```python
from build123d import *

# Parameters (mm, degrees)
SKETCH3_W           = 2.234278516
SKETCH3_H           = 3.869883908
BOSS_EXTRUDE1_DEPTH = 3.81
SKETCH4_W           = 2.234278516
SKETCH4_H           = 3.81
BOSS_EXTRUDE2_DEPTH = 1.27
SKETCH7_W           = 2.234278516
SKETCH7_H           = 3.81
BOSS_EXTRUDE3_DEPTH = 1.27
CUT_EXTRUDE3_DEPTH  = 2.286
FILLET1_R           = 0.254


with BuildPart() as part:
    # Sketch1 → Revolve1 (revolve)
    with BuildSketch(Plane.XY):
        with BuildLine():
            Line((0, 0), (6.604, 0))
            Line((6.604, 0), (6.604, 1.524))
            Line((6.604, 1.524), (5.526369265, 2.601630735))
            ThreePointArc((5.526369265, 2.601630735), (5.623645794, 3.729450681), (5.02050731, 4.687398762))
            Line((5.02050731, 4.687398762), (5.02050731, 6.211398762))
            add(Edge.make_bspline(
                [(5.02050731, 6.211398762), (2.796634976, 16.191993282), (2.733543957, 26.472012216)],
                knots=[0, 0, 0, 1, 1, 1], degree=2))
            Line((2.733543957, 26.472012216), (2.733543957, 31.552012216))
            ThreePointArc((2.733543957, 31.552012216), (3.551212648, 32.965759778), (2.300394609, 34.015863816))
            Line((2.300394609, 34.015863816), (2.300394609, 34.777863816))
            ThreePointArc((2.300394609, 34.777863816), (2.528411489, 35.490223347), (2.037352116, 36.054411694))
            add(Edge.make_bspline(
                [(2.037352116, 36.054411694), (2.754588802, 37.690610821), (3.171523279, 39.41712427), (3.279734912, 41.196512193)],
                knots=[0, 0, 0, 0, 0.825528863, 0.825528863, 0.825528863, 0.825528863], degree=3))
            ThreePointArc((3.279734912, 41.196512193), (3.026614336, 42.224230944), (2.234278516, 42.926))
            Line((2.234278516, 42.926), (0, 42.926))
            Line((0, 42.926), (0, 0))
        make_face()
    revolve(axis=Axis((0, 0, 0), (0, 1, 0)))

    # Sketch3 → Boss-Extrude1 (add)
    with BuildSketch(Plane(origin=(0, 42.926, 0), x_dir=(1, 0, 0), z_dir=(0, 1, 0))):
        Rectangle(SKETCH3_W, SKETCH3_H)
    extrude(amount=BOSS_EXTRUDE1_DEPTH)

    # Sketch4 → Boss-Extrude2 (add)
    with BuildSketch(Plane(origin=(0, 0, -1.934941954), x_dir=(-1, 0, 0), z_dir=(0, 0, -1))):
        with Locations((0, 44.831)):
            Rectangle(SKETCH4_W, SKETCH4_H)
    extrude(amount=BOSS_EXTRUDE2_DEPTH)

    # Sketch7 → Boss-Extrude3 (add)
    with BuildSketch(Plane.XY.offset(1.934941954)):
        with Locations((0, 44.831)):
            Rectangle(SKETCH7_W, SKETCH7_H)
    extrude(amount=BOSS_EXTRUDE3_DEPTH)

    # Sketch11 → Cut-Extrude3 (cut)
    with BuildSketch(Plane(origin=(1.117139258, 0, 0), x_dir=(0, 0, -1), z_dir=(1, 0, 0))):
        with BuildLine():
            Line((-1.934941954, 42.926), (-1.33813329, 42.926))
            Line((-1.33813329, 42.926), (-1.33813329, 43.942))
            ThreePointArc((-1.33813329, 43.942), (-1.412528167, 44.121605122), (-1.59213329, 44.196))
            Line((-1.59213329, 44.196), (-2.60813329, 44.196))
            ThreePointArc((-2.60813329, 44.196), (-2.787738412, 44.270394878), (-2.86213329, 44.45))
            Line((-2.86213329, 44.45), (-2.86213329, 45.212))
            ThreePointArc((-2.86213329, 45.212), (-2.787738412, 45.391605122), (-2.60813329, 45.466))
            Line((-2.60813329, 45.466), (-1.59213329, 45.466))
            ThreePointArc((-1.59213329, 45.466), (-1.412528167, 45.540394878), (-1.33813329, 45.72))
            Line((-1.33813329, 45.72), (-1.33813329, 46.10618983))
            Line((-1.33813329, 46.10618983), (-0.180981014, 46.680037288))
            ThreePointArc((-0.180981014, 46.680037288), (-0.06813329, 46.706482039), (0.044714435, 46.680037288))
            Line((0.044714435, 46.680037288), (1.20186671, 46.10618983))
            Line((1.20186671, 46.10618983), (1.20186671, 45.72))
            ThreePointArc((1.20186671, 45.72), (1.276261588, 45.540394878), (1.45586671, 45.466))
            Line((1.45586671, 45.466), (2.47186671, 45.466))
            ThreePointArc((2.47186671, 45.466), (2.651471833, 45.391605122), (2.72586671, 45.212))
            Line((2.72586671, 45.212), (2.72586671, 44.45))
            ThreePointArc((2.72586671, 44.45), (2.651471833, 44.270394878), (2.47186671, 44.196))
            Line((2.47186671, 44.196), (1.45586671, 44.196))
            ThreePointArc((1.45586671, 44.196), (1.276261588, 44.121605122), (1.20186671, 43.942))
            Line((1.20186671, 43.942), (1.20186671, 42.926))
            Line((1.20186671, 42.926), (1.934941954, 42.926))
            Line((1.934941954, 42.926), (3.204941954, 42.926))
            Line((3.204941954, 42.926), (3.204941954, 46.736))
            Line((3.204941954, 46.736), (-3.204941954, 46.736))
            Line((-3.204941954, 46.736), (-3.204941954, 42.926))
            Line((-3.204941954, 42.926), (-1.934941954, 42.926))
        make_face()
    extrude(amount=-CUT_EXTRUDE3_DEPTH, mode=Mode.SUBTRACT)

    # Fillet1
    fillet1_edges = [part.edges().sort_by_distance(p)[0] for p in [
        (0, 42.926, 1.33813329),
        (-1.117139258, 42.926, 0.06813329),
        (1.117139258, 42.926, 0.06813329),
        (0, 42.926, -1.20186671),
    ]]
    fillet(fillet1_edges, radius=FILLET1_R)


solid = part.part
```
CAD build for the part. Positions are in the model's coordinates, mm. A direction names the side the tool comes from. Coordinates: 2 decimals unless noted, no trailing zeros. Return JSON: item names as keys, results as strings.
1. Drop flat-ended pins along their axis: pin 1 (3 mm diameter, centred on y = 30, z = 3, fed in from +X); pin 2 (0.5 mm diameter, centred on x = 0.5, z = 2, fed in from +Y); pin 3 (1.3 mm diameter, centred on x = -0.5, z = -1, fed in from +Y). Give the stop position or say it passes through.
Result:
{"pin 1": "stops at x = 2.29", "pin 2": "stops at y = 45.47", "pin 3": "stops at y = 46.53"}
2. Probe L1, parallel to Y at x = 0.75, z = 2; L2, parallel to X at y = 24, z = -2; L3, parallel to Z at x = -0.75, y = 44.5. List the from-to ranges inside material, lowest first. Write a range as from..to.
Result:
{"L1": "y = 0..36.01, 36.28..42.93, 44.2..45.47", "L2": "x = -1.93..1.93", "L3": "z = -2.73..2.86"}
3. Mould opens along Y. For faces 1 (the flat face through (-1.117, 45, 0)), 2 (the flat face through (0, 45.466, 2)), 3 (the flat face through (0, 42.926, -2)), 4 (the flat face through (0, 44.196, -2)) say: released by +Y, released by -Y, zero draft, split by the parting line, or undercut.
Result:
{"face 1": "zero draft", "face 2": "released by +Y", "face 3": "undercut", "face 4": "undercut"}
4. 3-axis set-ups, long thin cutter, end or side, ignore diameter. For faces 5 (the flat face through (1.117, 45, 0)), 6 (the cylindrical face through (2.194, 34.402, -0.691)), 7 (the cylindrical face through (4.79, 5.46, -1.51)), 8 (the flat face through (0, 45.466, -2)), 9 (the flat face through (0, 44.196, 2)): which of +Z, -Z, +X, -X, +Y, -Y reach the whole face in a straight line?
Result:
{"face 5": "+Z, -Z, +X, +Y", "face 6": "none", "face 7": "+Y", "face 8": "-Z, +X, -X, +Y", "face 9": "+Z, +X, -X"}
